from build123d import *

# Parameters (mm, degrees)
SKETCH1_W            = 25
SKETCH1_H            = 25.4
BOSS_EXTRUDE1_DEPTH  = 6.8
SKETCH2_W            = 6.8
SKETCH2_H            = 15
BOSS_EXTRUDE2_DEPTH  = 6.8
FILLET1_R            = 3
FILLET1_OF_MIRROR1_R = 3
SKETCH3_R            = 2.125
CUT_EXTRUDE1_DEPTH   = 6.8


with BuildPart() as part:
    # Sketch1 → Boss-Extrude1 (new body)
    with BuildSketch(Plane.XY):
        Rectangle(SKETCH1_W, SKETCH1_H)
    extrude(amount=BOSS_EXTRUDE1_DEPTH)

    # Sketch2 → Boss-Extrude2 (add)
    with BuildSketch(Plane.XY.offset(6.8)):
        with Locations((15.9, 0)):
            Rectangle(SKETCH2_W, SKETCH2_H)
    boss_extrude2 = extrude(amount=-BOSS_EXTRUDE2_DEPTH)

    # Fillet1
    fillet1_edges = [part.edges().sort_by_distance(p)[0] for p in [
        (19.3, 7.5, 3.4),
        (19.3, -7.5, 3.4),
    ]]
    fillet(fillet1_edges, radius=FILLET1_R)

    # Mirror1: Boss-Extrude2 across plane
    add(boss_extrude2.mirror(Plane(origin=(0, 0, 0), x_dir=(0, 0, 1), z_dir=(1, 0, 0))))

    # Fillet1 of Mirror1
    fillet1_of_mirror1_edges = [part.edges().sort_by_distance(p)[0] for p in [
        (-19.3, 7.5, 3.4),
        (-19.3, -7.5, 3.4),
    ]]
    fillet(fillet1_of_mirror1_edges, radius=FILLET1_OF_MIRROR1_R)

    # Sketch3 → Cut-Extrude1 (cut)
    with BuildSketch(Plane.XY.offset(6.8)):
        Circle(SKETCH3_R)
    extrude(amount=-CUT_EXTRUDE1_DEPTH, mode=Mode.SUBTRACT)


solid = part.part
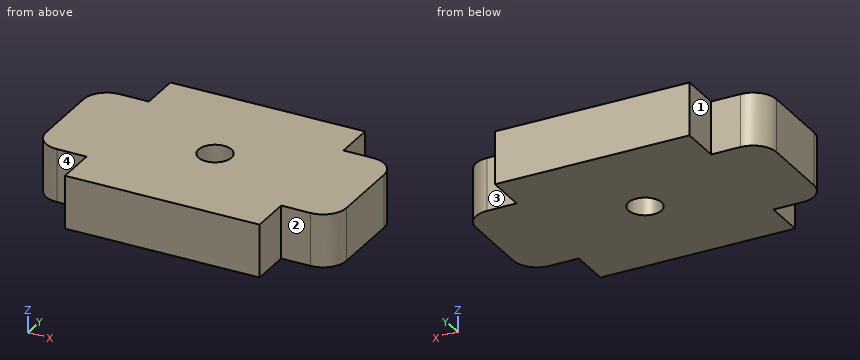
Work out the finished part from the listing and answer in its coordinate system (mm). Face numbers are marked on the shaded views. A direction names the side the tool comes from. Round coordinates to 2 decimals unless told otherwise and drop trailing zeros. Loops run counter-clockwise (first coordinate to the right, second up) from the corner with the lowest first, then second, coordinate; pieces in that order, holes last. Notation, with made-up numbers: (68, 8) - (111, 8) arc R19 cw to (111, 17) - close; hole circle Ø5 at (-3, 42.5). An arc over 180 degrees is marked (long way). Use one line per item in the form item = value. Start each with the question number.
(1) Flat-ended cylindrical pins translate along their axes: P1, Ø1.6, axis at y = -10, z = 3.5, coming from the +X side; P2, Ø4, axis at y = 10, z = 2, coming from the -X side; P3, Ø4, axis at y = 9, z = 4, coming from the +X side; P4, Ø1, axis at x = -1.5, y = -0.5, coming from the +Z side. Find the tip coordinate at first contact, or state that the pin passes through.
(2) Find section C-C on x = 0. Determine the outline of the cut face in (y, z) (3 decimals), and give its area (3 significant figures).
(3) Consider line 1 (Y direction, x = 0, z = 3.75) (3 decimals); line 2 (Y direction, x = 13.5, z = 5.5); line 3 (X direction, y = 11.5, z = 1.5). Determine where each line is inside the solid, lowest interval first.
(4) Find section B-B on z = 4. Determine the outline of the cut face in (x, y) (3 decimals), and give its area (3 significant figures).
(5) Find section D-D on y = 9. Determine the outline of the cut face in (x, z).
(6) Find section A-A on y = 0. Determine the outline of the cut face in (x, z) (3 decimals), and give its area (3 significant figures).
(7) Which of the six approach directions +Z, -Z, +X, -X, +Y, -Y give full straight-line access (tool end or side, diameter ignored) to the marked faces 1, 2, 3 and 4?
Answer list:
q1.P1 = 12.5
q1.P2 = -12.5
q1.P3 = 17.96
q1.P4 = through
q2.outline = (-12.7, 0) - (-2.125, 0) - (-2.125, 6.8) - (-12.7, 6.8) - close; (2.125, 0) - (12.7, 0) - (12.7, 6.8) - (2.125, 6.8) - close
q2.area = 144 mm^2
q3.line_1 = -12.7 to -2.125, 2.125 to 12.7
q3.line_2 = -7.5 to 7.5
q3.line_3 = -12.5 to 12.5
q4.outline = (-19.3, -4.5) arc R3 ccw to (-16.3, -7.5) - (-12.5, -7.5) - (-12.5, -12.7) - (12.5, -12.7) - (12.5, -7.5) - (16.3, -7.5) arc R3 ccw to (19.3, -4.5) - (19.3, 4.5) arc R3 ccw to (16.3, 7.5) - (12.5, 7.5) - (12.5, 12.7) - (-12.5, 12.7) - (-12.5, 7.5) - (-16.3, 7.5) arc R3 ccw to (-19.3, 4.5) - close; hole circle Ø4.25 at (0, 0)
q4.area = 817 mm^2
q5.outline = (-12.5, 0) - (12.5, 0) - (12.5, 6.8) - (-12.5, 6.8) - close
q6.outline = (-19.3, 0) - (-2.125, 0) - (-2.125, 6.8) - (-19.3, 6.8) - close; (2.125, 0) - (19.3, 0) - (19.3, 6.8) - (2.125, 6.8) - close
q6.area = 234 mm^2
q7.face_1 = +Z, -Z, -X, +Y
q7.face_2 = +Z, -Z, +X, -Y
q7.face_3 = +Z, -Z, +X, +Y
q7.face_4 = +Z, -Z, -X, -Y
